Could you check a few things on this model? Use its own coordinates, in mm. Face numbers are marked on the shaded views. A direction names the side the tool comes from. Give positions to 0.01 mm unless a question says otherwise; leave off trailing zeros. Loops run counter-clockwise (first coordinate to the right, second up) from the corner with the lowest first, then second, coordinate; pieces in that order, holes last.
1. Imagine slicing it at B-B (z = 24.5). List the corners of the cut face in (x, y) for me.
2. For P1, Ø3.5, axis at x = -8, z = 8.32, coming from the -Y side; P2, Ø9, axis at x = 8, y = -20, coming from the +Z side; P3, Ø4, axis at x = -3.5, z = 23, coming from the +Y side; P4, Ø4.5, axis at x = -7.5, y = -20.5, coming from the +Z side, each with a flat end and sliding along its axis, tell me the tip position at first contact or that it passes through.
3. Imagine slicing it at D-D (x = 12). List the corners of the cut face in (y, z) for me, plus the area to 3 significant figures.
4. I need wall thicknesses on line 1 along Y through (x, z) = (-8, 1.6); line 2 along X through (y, z) = (-20, 1.5); line 3 along X through (y, z) = (-20, 4.25). Which ranges of each line are inside material? Lowest first, please.
5. For the marked faces 1 and 2, which set-ups out of +Z, -Z, +X, -X, +Y, -Y let a thin tool reach every point of the face, with its end or its side?
6. Imagine slicing it at A-A (y = 20). List the corners of the cut face in (x, z) for me, plus the area to 3 significant figures.
7. Imagine slicing it at C-C (x = 8). Count the separate pieces of the cut face and the enclosed holes in it, plus the area to 3 significant figures.
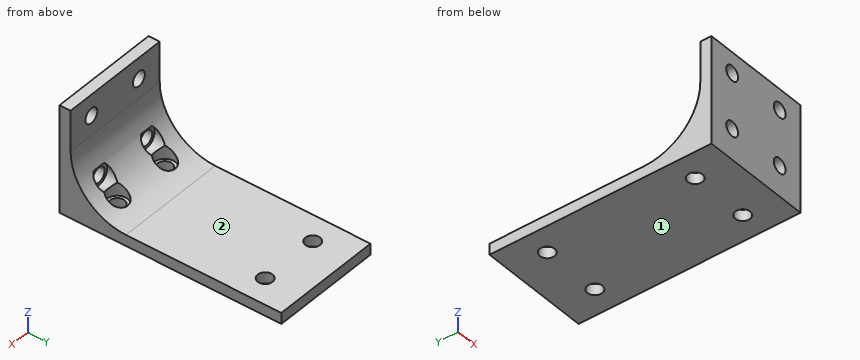
```python
from build123d import *

# Parameters (mm, degrees)
SKETCH1_W           = 30
SKETCH1_H           = 60
SKETCH1_R           = 2
BOSS_EXTRUDE1_DEPTH = 3
SKETCH2_W           = 26
SKETCH2_H           = 3
BOSS_EXTRUDE2_DEPTH = 15
SKETCH3_R           = 2
CUT_EXTRUDE1_DEPTH  = 66.6886596
FILLET1_R           = 15
CUT_EXTRUDE2_START  = 2
SKETCH4_R           = 2.8
CUT_EXTRUDE2_DEPTH  = 64.688659622
SKETCH5_R           = 2.8
CUT_EXTRUDE3_DEPTH  = 43.438190383


with BuildPart() as part:
    # Sketch1 → Boss-Extrude1 (new body)
    with BuildSketch(Plane.XY):
        Rectangle(SKETCH1_W, SKETCH1_H)
        with Locations((8, 20)):
            Circle(SKETCH1_R, mode=Mode.SUBTRACT)
        with Locations(Location((8, -20, 0), (0, 0, 180))):
            Circle(SKETCH1_R, mode=Mode.SUBTRACT)
        with Locations(Location((-8, 20, 0), (0, 0, 180))):
            Circle(SKETCH1_R, mode=Mode.SUBTRACT)
        with Locations((-8, -20)):
            Circle(SKETCH1_R, mode=Mode.SUBTRACT)
    extrude(amount=BOSS_EXTRUDE1_DEPTH)

    # Sketch2 → Boss-Extrude2 (add, symmetric)
    with BuildSketch(Plane(origin=(0, 0, 0), x_dir=(0, 0, -1), z_dir=(1, 0, 0))):
        with Locations((-16, -28.5)):
            Rectangle(SKETCH2_W, SKETCH2_H)
    extrude(amount=BOSS_EXTRUDE2_DEPTH, both=True)

    # Sketch3 → Cut-Extrude1 (cut, through all)
    with BuildSketch(Plane(origin=(0, -27, 0), x_dir=(1, 0, 0), z_dir=(0, 1, 0))):
        with Locations(Location((-8, -8.31541538, 0), (0, 0, 270))):
            Circle(SKETCH3_R)
        with Locations(Location((8, -8.31541538, 0), (0, 0, 270))):
            Circle(SKETCH3_R)
        with Locations(Location((-8, -23.31541538, 0), (0, 0, 270))):
            Circle(SKETCH3_R)
        with Locations(Location((8, -23.31541538, 0), (0, 0, 270))):
            Circle(SKETCH3_R)
    extrude(amount=-CUT_EXTRUDE1_DEPTH, mode=Mode.SUBTRACT)

    # Fillet1
    # the kernel refuses this fillet: 15 mm, written as the material it adds along each edge
    with BuildSketch(Plane(origin=(-15, -27, 3), x_dir=(0, 1, 0), z_dir=(1, 0, 0))) as fillet1_piece_1_section:
        with BuildLine():
            CenterArc((FILLET1_R, FILLET1_R), FILLET1_R, 180, 90)
            Line((0, FILLET1_R), (0, 0))
            Line((0, 0), (FILLET1_R, 0))
        make_face()
    fillet1_piece_1 = extrude(amount=30, mode=Mode.PRIVATE)
    fillet1_piece_1 = fillet1_piece_1 - Plane(origin=(-8, -20, 6.3866805), x_dir=(1, 0, 0), z_dir=(0, 0, -1)) * Cylinder(2, 120, mode=Mode.PRIVATE)
    fillet1_piece_1 = fillet1_piece_1 - Plane(origin=(8, -20, 6.3866805), x_dir=(-1, 0, 0), z_dir=(0, 0, -1)) * Cylinder(2, 120, mode=Mode.PRIVATE)
    fillet1_piece_1 = fillet1_piece_1 - Plane(origin=(-8, -23.64475421, 8.31541538), x_dir=(0, 0, 1), z_dir=(0, 1, 0)) * Cylinder(2, 120, mode=Mode.PRIVATE)
    fillet1_piece_1 = fillet1_piece_1 - Plane(origin=(8, -23.64475421, 8.31541538), x_dir=(0, 0, 1), z_dir=(0, 1, 0)) * Cylinder(2, 120, mode=Mode.PRIVATE)
    add(fillet1_piece_1)

    # Sketch4 → Cut-Extrude2 (cut, through all)
    with BuildSketch(Plane(origin=(0, -27, 0), x_dir=(1, 0, 0), z_dir=(0, 1, 0)).offset(CUT_EXTRUDE2_START)):
        with Locations((-8, -8.31541538)):
            Circle(SKETCH4_R)
        with Locations((8, -8.31541538)):
            Circle(SKETCH4_R)
    extrude(amount=CUT_EXTRUDE2_DEPTH, mode=Mode.SUBTRACT)

    # Sketch5 → Cut-Extrude3 (cut, through all)
    with BuildSketch(Plane.XY.offset(3)):
        with Locations(Location((-8, -20, 0), (0, 0, 218.180965893))):
            Circle(SKETCH5_R)
        with Locations(Location((8, -20, 0), (0, 0, 218.180965893))):
            Circle(SKETCH5_R)
    extrude(amount=CUT_EXTRUDE3_DEPTH, mode=Mode.SUBTRACT)


solid = part.part
```
Derived:
1. outline: (-15, -30) - (-9.61, -30) - (-9.61, -27) - (-15, -27) - close; (-6.39, -30) - (6.39, -30) - (6.39, -27) - (-6.39, -27) - close; (9.61, -30) - (15, -30) - (15, -27) - (9.61, -27) - close
2. P1: passes through
2. P2: stops at z = 8.4
2. P3: stops at y = -27
2. P4: stops at z = 6.7
3. outline: (-30, 0) - (30, 0) - (30, 3) - (-12, 3) arc R15 cw to (-27, 18) - (-27, 29) - (-30, 29) - close
3. area: 306 mm2
4. line 1: y = -30 to -22, -18 to 18, 22 to 30
4. line 2: x = -15 to -10, -6 to 6, 10 to 15
4. line 3: x = -15 to -10.8, -5.2 to 5.2, 10.8 to 15
5. face 1: -Z, +X, -X, +Y, -Y
5. face 2: +Z, +X, -X, +Y
6. outline: (-15, 0) - (-10, 0) - (-10, 3) - (-15, 3) - close; (-6, 0) - (6, 0) - (6, 3) - (-6, 3) - close; (10, 0) - (15, 0) - (15, 3) - (10, 3) - close
6. area: 66.0 mm2
7. separate pieces: 5
7. enclosed holes: 0
7. area: 229 mm2
